For this review, take the finished solid that the model builds, in its own axes (mm). A direction names the side the tool comes from. Coordinates: 2 decimals unless noted, no trailing zeros. Order: outer loops, then holes, each group sorted by start corner. A loop starts at its lowest first (then second) coordinate and runs counter-clockwise, first axis right, second up.
Autodesk Inventor part; units mm, degrees
ref_plane "Work Plane1" through (9.2625, 0, 0) normal (0, 0, 1) x (-1, 0, 0)
ref_plane "YZ Plane" through (0, 0, 0) normal (1, 0, 0) x (0, 1, 0)
ref_plane "XZ Plane" through (0, 0, 0) normal (0, 1, 0) x (-1, 0, 0)
sketch "Skizze1" plane through (0, 0, 0) normal (1, 0, 0) x (0, 1, 0)
  line L0 (1.5877, -2.75) -> (-1.5877, -2.75)
  line L1 (-1.5877, -2.75) -> (-3.1754, 0)
  line L2 (-3.1754, 0) -> (-1.5877, 2.75)
  line L3 (-1.5877, 2.75) -> (1.5877, 2.75)
  line L4 (1.5877, 2.75) -> (3.1754, 0)
  line L5 (3.1754, 0) -> (1.5877, -2.75)
  point P0 (0, 0)
  point P1 (0, 0)
  dimension "d0" = 6.3509
extrude "Körper" add sketch "Skizze1" along normal blind 1.55
sketch "Skizze2" plane through (1.55, 0, 0) normal (1, 0, 0) x (0, 0, -1)
  circle A0 centre (0, 0) radius 2.28
  dimension "d7" = 4.56
extrude "Ring" add sketch "Skizze2" along normal blind 2.35
sketch "Skizze3" plane through (0, 0, 0) normal (0, 0, 1) x (1, 0, 0)
  line L0 (0, 1.5877) -> (0, 3.1754)
  line L1 (0, 3.1754) -> (1.55, 3.1754)
  line L2 (1.55, 1.5877) -> (1.55, 3.1754)
  line L3 (-0.31, 0) -> (1.86, 0)
  line L4 (0, 2.28) -> (0.517, 3.1754)
  line L5 (1.033, 3.1754) -> (1.55, 2.28)
  dimension "d3" = 30
  dimension "d4" = 30
  dimension "d5" = 4.56
  dimension "d6" = 4.56
revolve "Fase1" cut sketch "Skizze3" angle 360 about axis through (-10, 0, 0) along (1, 0, 0)
sketch "Skizze4" plane through (0, 0, 0) normal (-1, 0, 0) x (0, 0, 1)
  line L0 (0, -4.4456) -> (0, 4.4456)
  line L1 (-3.85, 0) -> (3.85, 0)
  point P0 (0, 0)
hole "Gewinde" at (0, 0, 0) direction (1, 0, 0) diameter 2.459 end through all
chamfer "Fase2" distance 0.2706 angle 30 1 edges at (0, 0, -1.2295) measured on face at (0, 1.9048, -0.2313)
chamfer "Fase3" distance 0.2706 angle 30 1 edges at (3.9, 0, -1.2295) measured on face at (3.9, -0.28, -1.8958)
ref_plane "Work Plane1" through (9.2625, 0, 0) normal (0, 0, 1) x (-1, 0, 0)
equation "\"d0\" = 1.1547 * SW"
equation "\"d1\" = KOH1"
equation "\"d7\" = SD2"
equation "\"d8\" = KOH - KOH1"
equation "\"d3\" = ANG1"
equation "\"d4\" = ANG2"
equation "\"d5\" = SW0"
equation "\"d6\" = SW01"
equation "\"d10\" = -0.5 * GD1 + 0.5 * NND"
equation "\"d46\" = -0.5 * GD1 + 0.5 * NND"
equation "\"d12\" = -0.5 * GD1 + 0.5 * NND"
equation "\"d47\" = -0.5 * GD1 + 0.5 * NND"
equation "\"ANG1\" = 30deg"
equation "\"ANG2\" = 30deg"
equation "\"NND\" = 3"
equation "\"KOH1\" = 1.55"
equation "\"KOH\" = 3.9"
equation "\"SW\" = 5.5"
equation "\"SW0\" = 4.56"
equation "\"SW01\" = SW0"
equation "\"SD2\" = SW0"
equation "\"GUL\" = 0.541266 * PTC"
equation "\"THREADDIA\" = 3"
equation "\"TOA\" = 30deg"
equation "\"PTC\" = 0.5"
equation "\"E0\" = 1.155 * SW"
equation "\"GAL\" = 0.541266 * PTC"
properties part number "ISO 10511 - M3" material "Stahl, weich"
1. Clearance check with flat-ended pins moving along their axes: pin 1 Ø1.5 at (x, z) = (3.5, 1.5) entering from -Y; pin 2 Ø1.5 at (x, y) = (3.5, 1.5) entering from +Z. State where each tip first meets the part, or that it passes through.
Answer below:
pin 1: stops at y = -2.15
pin 2: stops at z = 2.15
2. Take a section at B-B, the plane x = 2.8. Give the boundary of the cut face in (y, z).
Answer below:
outline: circle Ø4.56 at (0, 0); hole circle Ø2.46 at (0, 0)
3. Machinability: for faces 1 (the face through (2.7, 1.4, 1.8)), 2 (the face through (1, 0, -2.75)), which of the approach directions +Z, -Z, +X, -X, +Y, -Y give a long, thin tool a straight path to every point of the face, cutting with its end or side? Answer none if there is none.
Answer below:
face 1: +X
face 2: -Z, +X, -X, +Y, -Y
4. Take a section at A-A, the plane y = 0. Give the boundary of the cut face in (x, z), plus the area to 3 significant figures.
Answer below:
outline: (0, -2.28) - (0.27, -2.75) - (1.28, -2.75) - (1.55, -2.28) - (3.9, -2.28) - (3.9, -1.5) - (3.74, -1.23) - (0.16, -1.23) - (0, -1.5) - close; (0, 1.5) - (0.16, 1.23) - (3.74, 1.23) - (3.9, 1.5) - (3.9, 2.28) - (1.55, 2.28) - (1.28, 2.75) - (0.27, 2.75) - (0, 2.28) - close
area: 9.31 mm2
5. To check wall thickness, follow L1, parallel to Y at x = 2.8, z = 0; L2, parallel to Y at x = 1.1, z = 0.7. State the ranges of each line that lie inside material, in increasing order.
Answer below:
L1: y = -2.28 to -1.23, 1.23 to 2.28
L2: y = -2.77 to -1.01, 1.01 to 2.77
